from build123d import *

# Parameters (mm, degrees)
SCHIZZO1_R                   = 2.485
ESTRUSIONE_ESTRUSIONE1_DEPTH = 11.9
ESTRUSIONE_ESTRUSIONE2_START = -2.485
ESTRUSIONE_ESTRUSIONE2_DEPTH = 4.97
SCHIZZO3_R                   = 1.98
TAGLIO_ESTRUSIONE1_DEPTH     = 15.757761517
SCHIZZO4_R                   = 1.05
TAGLIO_ESTRUSIONE2_DEPTH     = 15.116155638
TAGLIO_ESTRUSIONE3_START     = -1.5
SCHIZZO5_R                   = 3.035
TAGLIO_ESTRUSIONE3_DEPTH     = 1.5


# Read off the part's stored shape, not the designer's step: Estrusione-Estrusione2
with BuildPart() as part:
    # Schizzo1 → Estrusione-Estrusione1 (new body)
    with BuildSketch(Plane(origin=(0, 0, 0), x_dir=(0, 0, -1), z_dir=(1, 0, 0))):
        Circle(SCHIZZO1_R)
    extrude(amount=ESTRUSIONE_ESTRUSIONE1_DEPTH)

    # Estrusione-Estrusione2 outline → Estrusione-Estrusione2 (add)
    with BuildSketch(Plane(origin=(0, 0, 0), x_dir=(1, 0, 0), z_dir=(0, 1, 0)).offset(ESTRUSIONE_ESTRUSIONE2_START)):
        with BuildLine():
            Line((8.985, 0), (8.985, 4.14))
            ThreePointArc((8.985, 4.14), (5.95, 7.175), (2.915, 4.14))
            Line((2.915, 4.14), (2.915, 0))
            Line((2.915, 0), (8.985, 0))
        make_face()
    extrude(amount=ESTRUSIONE_ESTRUSIONE2_DEPTH)

    # Schizzo3 → Taglio-Estrusione1 (cut, through all)
    with BuildSketch(Plane(origin=(0, 2.485, 0), x_dir=(1, 0, 0), z_dir=(0, 1, 0))):
        with Locations(Location((5.95, 4.14, 0), (0, 0, 270))):
            Circle(SCHIZZO3_R)
    extrude(amount=-TAGLIO_ESTRUSIONE1_DEPTH, mode=Mode.SUBTRACT)

    # Schizzo4 → Taglio-Estrusione2 (cut, through all)
    with BuildSketch(Plane.ZY):
        Circle(SCHIZZO4_R)
    extrude(amount=-TAGLIO_ESTRUSIONE2_DEPTH, mode=Mode.SUBTRACT)

    # Schizzo5 → Taglio-Estrusione3 (cut)
    with BuildSketch(Plane(origin=(0, 2.485, 0), x_dir=(1, 0, 0), z_dir=(0, 1, 0)).offset(TAGLIO_ESTRUSIONE3_START)):
        with Locations((5.95, 4.14)):
            Circle(SCHIZZO5_R)
    extrude(amount=TAGLIO_ESTRUSIONE3_DEPTH, mode=Mode.SUBTRACT)


solid = part.part
Can you work these out from the model? Positions are in its coordinate system, mm. A direction names the side the tool comes from. Coordinates: 2 decimals unless noted, no trailing zeros. Order: outer loops, then holes, each group sorted by start corner. A loop starts at its lowest first (then second) coordinate and runs counter-clockwise, first axis right, second up. Notation, with made-up numbers: (16, -12) - (38, -12) arc R21 ccw to (38, 12) - close; hole circle Ø7 at (1, -34). An arc over 180 degrees is marked (long way). Answer as a JSON object with one key per item and string values. Group by question number.
Q1. Imagine slicing it at B-B (x = 5.95). Please give me the cut outline in (y, z) (3 decimals), and give its area (4 significant figures).
Q2. Imagine slicing it at C-C (z = -5). Please give me the cut outline in (x, y) (3 decimals), and give its area (3 significant figures).
Q3. Imagine slicing it at D-D (y = -2.1). Please give me the cut outline in (x, z) (3 decimals), and give its area (3 significant figures).
Q4. I need wall thicknesses on line 1 (Y direction, x = 5.75, z = 0) (3 decimals); line 2 (X direction, y = -1.45, z = -4.14) (3 decimals); line 3 (Z direction, x = 7.75, y = -0.3). Which ranges of each line are inside material? Lowest first, please. Write a range as from..to.
Q5. On a 3-axis mill with a long thin cutter (end or side, diameter ignored), from which of +Z, -Z, +X, -X, +Y, -Y can I reach the whole of each face in a straight line? I mean faces 4 (the face through (5.867, 0.109, 2.483)), 5 (the face through (5.883, 1.724, -1.106)), 6 (the face through (6.017, -0.774, -7.174)). Say none if no direction works.
Q6. Will these pins go through, and if not, where does the flat tip stop? P1, Ø1, axis at x = 7, z = -5.5, coming from the +Y side (3 decimals); P2, Ø1, axis at y = 0.5, z = -3, coming from the +X side (3 decimals); P3, Ø1, axis at x = 6.5, z = -3, coming from the +Y side.
Q7. Imagine slicing it at A-A (y = -0.85). Please give me the cut outline in (x, z) (3 decimals).
Q8. We'd pull the mould along X, two halves only. Please class faces 1 (the face through (2.915, 0, -3)), 2 (the face through (6, 0.985, -2)), 3 (the face through (6, -2.485, -2)): +X half, -X half, draft (parallel to the pull), parting line (faces both ways), or undercut.
Determined:
{
 "1": {"outline": "(-2.485, -7.175) - (0.985, -7.175) - (0.985, -6.12) - (-2.485, -6.12) - close; (-2.485, -2.16) - (0.985, -2.16) - (0.985, -1.105) - (2.485, -1.105) - (2.485, 0) arc R2.485 ccw to (-2.485, 0) - close; hole circle Ø2.1 at (0, 0)", "area": "19.05 mm2"},
 "2": {"outline": "(3.039, -2.485) - (4.167, -2.485) - (4.167, 0.985) - (3.039, 0.985) - close; (7.733, -2.485) - (8.861, -2.485) - (8.861, 0.985) - (7.733, 0.985) - close", "area": "7.82 mm2"},
 "3": {"outline": "(0, -1.329) - (2.915, -1.329) - (2.915, -4.14) arc R3.035 ccw to (8.985, -4.14) - (8.985, -1.329) - (11.9, -1.329) - (11.9, 1.329) - (0, 1.329) - close; hole circle Ø3.96 at (5.95, -4.14)", "area": "50.8 mm2"},
 "4": {"line 1": "y = -2.485..-1.05, 1.05..2.485", "line 2": "x = 2.915..3.97, 7.93..8.985", "line 3": "z = -6.58..-4.96, -3.32..-1.01, 1.01..2.47"},
 "5": {"face 4": "none", "face 5": "-Z, +Y", "face 6": "-Z, +Y, -Y"},
 "6": {"P1": "stops at y = 0.985", "P2": "stops at x = 8.985", "P3": "passes through"},
 "7": {"outline": "(0, -2.335) - (2.915, -2.335) - (2.915, -4.14) arc R3.035 ccw to (8.985, -4.14) - (8.985, -2.335) - (11.9, -2.335) - (11.9, -0.616) - (0, -0.616) - close; (0, 0.616) - (11.9, 0.616) - (11.9, 2.335) - (0, 2.335) - close; hole circle Ø3.96 at (5.95, -4.14)"},
 "8": {"face 1": "-X half", "face 2": "undercut", "face 3": "draft"}
}
